Can you work these out from the model? Positions are in its coordinate system, mm. A direction names the side the tool comes from. Coordinates: 2 decimals unless noted, no trailing zeros. Write each loop counter-clockwise with the first axis right and the second up, starting at its lowest first coordinate (ties: lowest second). Pieces come first, ordered by that corner, then holes. Notation, with made-up numbers: M 14.5,85.25 L 58.5,85.25 A16 ccw 58.5,100.25 Z; hole C -33.75,89.25 d4. An arc over 180 degrees is marked long. Answer as a JSON object with one key per item and string values. Group by question number.
from build123d import *

# Parameters (mm, degrees)
ESQUISSE1_R                                = 30
BOSS_EXTRU_1_DEPTH                         = 15
ESQUISSE2_R                                = 12.5
BOSS_EXTRU_2_DEPTH                         = 69
ESQUISSE4_2_W                              = 230
ESQUISSE4_2_H                              = 40
ENL_V_MAT_EXTRU_1_DEPTH                    = 5
CHAMBRAGE_POUR_VIS_T_TE_HEXAGONALE_2_COUNT = 2
CHAMBRAGE_POUR_VIS_T_TE_HEXAGONALE_2_PITCH = 41
ESQUISSE17_R                               = 6
BOSS_EXTRU_4_DEPTH                         = 55


with BuildPart() as part:
    # Esquisse1 → Boss.-Extru.1 (new body)
    with BuildSketch(Plane.XY):
        Circle(ESQUISSE1_R)
    extrude(amount=BOSS_EXTRU_1_DEPTH)

    # Esquisse2 → Boss.-Extru.2 (add)
    with BuildSketch(Plane(origin=(0, 0, 0), x_dir=(-1, 0, 0), z_dir=(0, 0, -1))):
        with Locations(Location((0, 0, 0), (0, 0, 180))):
            Circle(ESQUISSE2_R)
    extrude(amount=BOSS_EXTRU_2_DEPTH)

    # Esquisse4_2 → Enl_v. mat.-Extru.1 (cut)
    with BuildSketch(Plane.XY.offset(15)):
        Rectangle(ESQUISSE4_2_W, ESQUISSE4_2_H)
    extrude(amount=-ENL_V_MAT_EXTRU_1_DEPTH, mode=Mode.SUBTRACT)

    # Esquisse14 → Chambrage pour vis _ t_te hexagonale M51 (revolve, cut)
    with BuildSketch(Plane.YZ.offset(-20.5)):
        Polygon((0, 0), (0, 15), (2.75, 15), (2.75, 3.605), (2.775, 3.58), (6.12, 3.58), (6.12, 0), align=None)
    chambrage_pour_vis_t_te_hexagonale_m51 = revolve(axis=Axis((-20.5, 0, -6.35), (0, 0, 1)), mode=Mode.SUBTRACT)

    # Chambrage pour vis _ t_te hexagonale 2: Chambrage pour vis _ t_te hexagonale M51 ×2
    with Locations(*[(i * CHAMBRAGE_POUR_VIS_T_TE_HEXAGONALE_2_PITCH, 0, 0) for i in range(1, CHAMBRAGE_POUR_VIS_T_TE_HEXAGONALE_2_COUNT)]):
        add(chambrage_pour_vis_t_te_hexagonale_m51, mode=Mode.SUBTRACT)

    # Esquisse17 → Boss.-Extru.4 (add)
    with BuildSketch(Plane(origin=(0, 0, -69), x_dir=(-1, 0, 0), z_dir=(0, 0, -1))):
        Circle(ESQUISSE17_R)
    extrude(amount=BOSS_EXTRU_4_DEPTH)


solid = part.part
Q1. Please list where these lines run through material, in increasing order: L1, parallel to X at y = 0, z = 2.3; L2, parallel to X at y = 0, z = 7; L3, parallel to Z at x = -27, y = -7.5.
Q2. If we section it at D-D on z = 5.5: List the corners of the cut face in (x, y) for me.
Q3. We'd pull the mould along Y, two halves only. Please class faces 1 (the cylindrical face through (-3.905, 29.745, 5.728)), 2 (the flat face through (0, 0, -124)), 3 (the flat face through (0, 0, 10)): pulls with the +Y half, pulls with the -Y half, needs draft (parallel to the pull), parting line crosses it, or undercut.
Q4. Will these pins go through, and if not, where does the flat tip stop? pin 1 (2.5 mm diameter, centred on x = 1.5, z = 13.5, fed in from +Y); pin 2 (9 mm diameter, centred on x = 20.5, y = 0, fed in from -Z); pin 3 (12 mm diameter, centred on x = 13.5, z = -25.5, fed in from +Y); pin 4 (6 mm diameter, centred on y = -17.5, z = -9.5, fed in from -X).
Q5. If we section it at C-C on x = -20.5: List the corners of the cut face in (y, z) for me (3 decimals).
Q6. On a 3-axis mill with a long thin cutter (end or side, diameter ignored), from which of +Z, -Z, +X, -X, +Y, -Y can I reach the whole of each face in a straight line? I mean faces 4 (the flat face through (0, 24, 15)), 5 (the cylindrical face through (6, 0, -96)), 6 (the flat face through (0, -20, 13)). Say none if no direction works.
Q7. If we section it at A-A on y = 0: Give the number of separate pieces and of enclosed holes in the cut face, and give its area (3 significant figures).
Q8. If we section it at B-B on x = 0: List the corners of the cut face in (y, z) for me.
Reply:
{
 "1": {"L1": "-30 to -26.62, -14.38 to 14.38, 26.62 to 30", "L2": "-30 to -23.25, -17.75 to 17.75, 23.25 to 30", "L3": "0 to 10"},
 "2": {"outline": "C 0,0 d60; hole C -20.5,0 d5.5; hole C 20.5,0 d5.5"},
 "3": {"face 1": "parting line crosses it", "face 2": "needs draft", "face 3": "undercut"},
 "4": {"pin 1": "y = 30", "pin 2": "z = 3.58", "pin 3": "y = 10", "pin 4": "through"},
 "5": {"outline": "M -21.903,0 L -6.12,0 L -6.12,3.58 L -2.775,3.58 L -2.75,3.605 L -2.75,10 L -20,10 L -20,15 L -21.903,15 Z; M 2.75,3.605 L 2.775,3.58 L 6.12,3.58 L 6.12,0 L 21.903,0 L 21.903,15 L 20,15 L 20,10 L 2.75,10 Z"},
 "6": {"face 4": "+Z, +X, -X, +Y, -Y", "face 5": "-Z", "face 6": "+Z, +X, -X"},
 "7": {"separate pieces": "3", "enclosed holes": "0", "area": "2,830 mm^2"},
 "8": {"outline": "M -30,0 L -12.5,0 L -12.5,-69 L -6,-69 L -6,-124 L 6,-124 L 6,-69 L 12.5,-69 L 12.5,0 L 30,0 L 30,15 L 20,15 L 20,10 L -20,10 L -20,15 L -30,15 Z"}
}
